Can you work these out from the model? Positions are in its coordinate system, mm. A direction names the side the tool comes from. Give positions to 0.01 mm unless a question says otherwise; leave off trailing zeros. Loops run counter-clockwise (first coordinate to the right, second up) from the corner with the lowest first, then second, coordinate; pieces in that order, holes last. Notation, with made-up numbers: (50, -32.5) - (87, -32.5) arc R14 cw to (87, -5.5) - close; hole circle Ø5 at (60.25, -2). An arc over 180 degrees is marked (long way). Use a Markdown table: item, result. Add a question column.
```python
from build123d import *

# Parameters (mm, degrees)
F1_DEPTH = 25


# Not quite as in the source:
# - ends of sketch curves that miss each other by under 0.0002 mm in the source are joined


with BuildPart() as f1:
    # F0 (on Top) → F1 (new body)
    with BuildSketch(Plane.XY):
        with BuildLine():
            ThreePointArc((-82.6844, 0), (0, -82.6844), (82.6844, 0))
            ThreePointArc((82.6844, 0), (0, 82.6844), (-82.6844, 0))
        make_face()
        with BuildLine():
            ThreePointArc((-0.0001019994, -64.3575904446), (-8.9899783863, -63.7364917021), (-17.8043990333, -61.8630911161))
            Line((-17.8043990333, -61.8630911161), (0, -22.3774))
            Line((0, -22.3774), (17.7835, -61.8695))
            ThreePointArc((17.7835, -61.8695), (8.9783061535, -63.7325605397), (-0.0001019994, -64.3575904446))
        make_face(mode=Mode.SUBTRACT)
        with BuildLine():
            ThreePointArc((-64.3576040742, 5e-06), (-63.8166972636, 8.3999218175), (-62.181104878, 16.6567989674))
            Line((-62.181104878, 16.6567989674), (-28.7278, -57.6069))
            ThreePointArc((-28.7278, -57.6069), (-54.7289693105, -33.866650173), (-64.3576040742, 5e-06))
        make_face(mode=Mode.SUBTRACT)
        with BuildLine():
            ThreePointArc((64.356106725, 9e-06), (54.7239343065, -33.864451622), (28.7263060265, -57.6068980531))
            Line((28.7263060265, -57.6068980531), (62.2183, 16.5153))
            ThreePointArc((62.2183, 16.5153), (63.8186125658, 8.3264340159), (64.356106725, 9e-06))
        make_face(mode=Mode.SUBTRACT)
        with BuildLine():
            Line((0, 21.6991), (-18.1035, 61.7762))
            ThreePointArc((-18.1035, 61.7762), (-9.143995, 63.7130624999), (-9.9e-05, 64.355997063))
            ThreePointArc((-9.9e-05, 64.355997063), (9.132463164, 63.7090225476), (18.0825989725, 61.7810009054))
            Line((18.0825989725, 61.7810009054), (0, 21.6991))
        make_face(mode=Mode.SUBTRACT)
        with BuildLine():
            Line((10.9234, 1.7325), (34.545, 54.3084))
            ThreePointArc((34.545, 54.3084), (44.0251133087, 46.9417504609), (51.9809939632, 37.9504079731))
            Line((51.9809939632, 37.9504079731), (22.3019, -27.7266))
            Line((22.3019, -27.7266), (10.8496, -2.2616))
            Line((10.8496, -2.2616), (-10.8494, -2.2616))
            Line((-10.8494, -2.2616), (-22.3016, -27.7266))
            Line((-22.3016, -27.7266), (-51.9378, 38.0118))
            ThreePointArc((-51.9378, 38.0118), (-44.0003546147, 46.9677472651), (-34.5479019666, 54.3069079476))
            Line((-34.5479019666, 54.3069079476), (-10.8494, 1.7325))
            Line((-10.8494, 1.7325), (10.9234, 1.7325))
        make_face(mode=Mode.SUBTRACT)
    extrude(amount=F1_DEPTH)


solid = f1.part
```
1. Suppose I cut it at A-A (z = 19.75). List the corners of the cut face in (x, y) for me (1 decimal), and give its area (3 significant figures).
2. Suppose I cut it at D-D (y = -53). List the corners of the cut face in (x, z) for me, and give its area (3 significant figures).
3. If we mould it in two halves opening along Y, with no side actions, what happens to faces 1 (the face through (-17.92, -80.72, 12.32)), 2 (the face through (-36.91, 4.68, 12.32)), 3 (the face through (-1, -17, 0))? For each: released by +Y, released by -Y, zero draft, split by the parting line, or undercut.
4. Suppose I cut it at C-C (x = -58.5). List the corners of the cut face in (y, z) for me, and give its area (3 significant figures).
5. Suppose I cut it at B-B (y = 41). List the corners of the cut face in (x, z) for me.
6. Will these pins go through, and if not, where does the flat tip stop? P1, Ø3, axis at y = 23, z = 14.5, coming from the -X side; P2, Ø6.5, axis at x = 2.5, z = 11.5, coming from the -Y side; P3, Ø5, axis at x = -43, z = 3, coming from the -Y side.
7. Please list where these lines run through material, in increasing order: line 1 along Y through (x, z) = (-1.5, 21.5); line 2 along Y through (x, z) = (-36, 19.5); line 3 along Y through (x, z) = (50, 22.75). Write a range as [from, to].
8. On a 3-axis mill with a long thin cutter (end or side, diameter ignored), from which of +Z, -Z, +X, -X, +Y, -Y can I reach the whole of each face in a straight line? I mean faces 4 (the face through (-1, -17, 25)), 5 (the face through (-8.925, 41.457, 12.325)). Say none if no direction works.
Results below:
| question | item | result |
|---|---|---|
| 1 | outline | circle Ø165.4 at (0, 0); hole (-64.4, 0) arc R64.4 ccw to (-28.7, -57.6) - (-62.2, 16.7) arc R64.2 ccw to start; hole (-51.9, 38) - (-22.3, -27.7) - (-10.8, -2.3) - (10.8, -2.3) - (22.3, -27.7) - (52, 38) arc R64.7 ccw to (34.5, 54.3) - (10.9, 1.7) - (-10.8, 1.7) - (-34.5, 54.3) arc R64.6 ccw to start; hole (-18.1, 61.8) - (0, 21.7) - (18.1, 61.8) arc R64.8 ccw to (0, 64.4) arc R64.3 ccw to start; hole (-17.8, -61.9) arc R64.2 ccw to (0, -64.4) arc R64.8 ccw to (17.8, -61.9) - (0, -22.4) - close; hole (28.7, -57.6) arc R64.4 ccw to (64.4, 0) arc R65 ccw to (62.2, 16.5) - close |
| 1 | area | 15,200 mm² |
| 2 | outline | (-63.46, 0) - (-36.53, 0) - (-36.53, 25) - (-63.46, 25) - close; (-30.8, 0) - (-13.81, 0) - (-13.81, 25) - (-30.8, 25) - close; (13.79, 0) - (30.81, 0) - (30.81, 25) - (13.79, 25) - close; (36.52, 0) - (63.46, 0) - (63.46, 25) - (36.52, 25) - close |
| 2 | area | 2,200 mm² |
| 3 | face 1 | split by the parting line |
| 3 | face 2 | undercut |
| 3 | face 3 | zero draft |
| 4 | outline | (-58.43, 0) - (-26.83, 0) - (-26.83, 25) - (-58.43, 25) - close; (8.49, 0) - (58.43, 0) - (58.43, 25) - (8.49, 25) - close |
| 4 | area | 2,040 mm² |
| 5 | outline | (-71.8, 0) - (-49.61, 0) - (-49.61, 25) - (-71.8, 25) - close; (-28.55, 0) - (-8.72, 0) - (-8.72, 25) - (-28.55, 25) - close; (8.71, 0) - (28.57, 0) - (28.57, 25) - (8.71, 25) - close; (49.61, 0) - (71.8, 0) - (71.8, 25) - (49.61, 25) - close |
| 6 | P1 | x = -79.84 |
| 6 | P2 | y = -82.68 |
| 6 | P3 | y = -72.09 |
| 7 | line 1 | [-82.67, -64.34], [-25.7, -2.26], [1.73, 25.02], [64.34, 82.67] |
| 7 | line 2 | [-74.44, -53.36], [-41.46, 2.66], [53.35, 74.44] |
| 7 | line 3 | [-65.85, -40.52], [-10.53, 33.57], [40.52, 65.85] |
| 8 | face 4 | +Z, +X, -X, +Y, -Y |
| 8 | face 5 | +Z, -Z |
